Model file for the job. Use its own axes, mm. A direction names the side the tool comes from. Give positions to 0.01 mm unless a question says otherwise; leave off trailing zeros. Order: outer loops, then holes, each group sorted by start corner. A loop starts at its lowest first (then second) coordinate and runs counter-clockwise, first axis right, second up. Notation, with made-up numbers: (81, 0.5) -> (102, 0.5) arc R5 cw to (102, 9.5) -> close; hole circle Ø5 at (41.5, -37). An arc over 180 degrees is marked (long way). Answer in a Markdown table with one row per item. Add a question column.
Autodesk Inventor part; units mm, degrees
ref_plane "Work Plane1" through (0, 0, 18.4) normal (0, 0, -1) x (-1, 0, 0)
ref_plane "YZ Plane" through (0, 0, 0) normal (1, 0, 0) x (0, 1, 0)
ref_plane "XZ Plane" through (0, 0, 0) normal (0, 1, 0) x (-1, 0, 0)
sketch "Sketch1" plane through (0, 0, 0) normal (0, 0, 1) x (1, 0, 0)
  line L0 (-11.5182, 8.1773) -> (10.9818, 8.1773)
  line L1 (10.9818, 8.1773) -> (10.9818, -3.6227)
  line L2 (10.9818, -3.6227) -> (-11.5182, -3.6227)
  line L3 (-11.5182, -3.6227) -> (-11.5182, 8.1773)
  point P0 (0, 0)
  dimension "d0" = 22.5
  dimension "d1" = 11.8
extrude "Extrusion1" add sketch "Sketch1" along normal blind 22.7
sketch "Sketch2" plane through (0, 0, 22.7) normal (0, 0, 1) x (1, 0, 0)
  arc A0 (-0.2741, 4.7773) -> (-0.2741, -0.2227) centre (-5.6182, 2.2773) ccw
  line L0 (-11.5182, 8.1773) -> (-11.5182, -3.6227)
  line L1 (-11.5182, -3.6227) -> (10.9818, -3.6227)
  line L2 (-0.2741, 4.7773) -> (0.6818, 4.7773)
  line L3 (0.6818, -0.2227) -> (-0.2741, -0.2227)
  arc A1 (0.6818, -0.2227) -> (0.6818, 4.7773) centre (0.6818, 2.2773) ccw
  line L4 (3.1818, 2.2773) -> (3.1818, 4.4746) construction
  point P0 (0, 0)
  dimension "d4" = 11.8
  dimension "d5" = 5.9
  dimension "d6" = 5
  dimension "d7" = 8.8
  dimension "d8" = 2.5
extrude "Extrusion2" add sketch "Sketch2" along normal blind 4 contours L2 A1 L3 A0
sketch "Sketch3" plane through (0, 0, 26.7) normal (0, 0, 1) x (1, 0, 0)
  line L0 (0.6818, 4.7773) -> (-0.2741, 4.7773)
  arc A0 (-0.2741, 4.7773) -> (-0.2741, -0.2227) centre (-5.6182, 2.2773) ccw
  line L1 (-0.2741, -0.2227) -> (0.6818, -0.2227)
  arc A1 (0.6818, -0.2227) -> (0.6818, 4.7773) centre (0.6818, 2.2773) ccw
  circle A2 centre (-5.6182, 2.2773) radius 2.3
  point P0 (0, 0)
  dimension "d11" = 4.6
extrude "Extrusion3" add sketch "Sketch3" along normal blind 3.2 contours A2
ref_plane "Work Plane1" through (0, 0, 18.4) normal (0, 0, -1) x (-1, 0, 0)
sketch "Sketch4" plane through (0, 0, 18.4) normal (0, 0, -1) x (-1, 0, 0)
  line L0 (11.5182, 8.1773) -> (-10.9818, 8.1773)
  line L1 (-10.9818, 8.1773) -> (-10.9818, -3.6227)
  line L2 (-10.9818, -3.6227) -> (11.5182, -3.6227)
  line L3 (11.5182, -3.6227) -> (11.5182, 8.1773)
  line L4 (11.5182, 8.1773) -> (16.2182, 8.1773)
  line L5 (16.2182, 8.1773) -> (16.2182, -3.6227)
  line L6 (16.2182, -3.6227) -> (11.5182, -3.6227)
  line L7 (11.5182, -3.6227) -> (11.5182, 8.1773)
  line L8 (-10.9818, 8.1773) -> (-15.6818, 8.1773)
  line L9 (-15.6818, 8.1773) -> (-15.6818, -3.6227)
  line L10 (-15.6818, -3.6227) -> (-10.9818, -3.6227)
  line L11 (-10.9818, -3.6227) -> (-10.9818, 8.1773)
  arc A0 (14.6782, 2.9273) -> (14.6782, 1.6273) centre (13.9182, 2.2773) ccw
  arc A1 (-14.1417, 1.6273) -> (-14.1417, 2.9273) centre (-13.3818, 2.2773) ccw
  line L12 (-14.1417, 2.9273) -> (-15.6818, 2.9273)
  line L13 (-14.1417, 1.6273) -> (-15.6818, 1.6273)
  line L14 (16.2182, 2.9273) -> (14.6782, 2.9273)
  line L15 (16.2182, 1.6273) -> (14.6782, 1.6273)
  point P0 (0, 0)
  dimension "d15" = 4.7
  dimension "d16" = 4.7
  dimension "d17" = 5.9
  dimension "d18" = 5.9
  dimension "d19" = 2
  dimension "d20" = 2
  dimension "d23" = 2.3
  dimension "d24" = 2.3
  dimension "d25" = 1.3
  dimension "d26" = 1.3
  dimension "d27" = 0.65
  dimension "d28" = 0.65
extrude "Extrusion4" add sketch "Sketch4" along normal blind 2.5 contours L4 L5 L14 A0 L15 L6 L3 | L1 L10 L9 L13 A1 L12 L8
sketch "Sketch5" plane through (-11.5182, -3.6227, 0) normal (-1, 0, 0) x (0, 0, 1)
  line L0 (5.7, 7.7) -> (4.5, 7.7)
  line L1 (4.5, 7.7) -> (4.5, 4.1)
  line L2 (4.5, 4.1) -> (5.7, 4.1)
  line L3 (5.7, 4.1) -> (5.7, 7.7)
  line L4 (0, 0) -> (0, 11.8)
  line L5 (0, 5.9) -> (2.0483, 5.9) construction
  point P0 (0, 3.6227)
  dimension "d31" = 1.2
  dimension "d32" = 3.6
  dimension "d33" = 4.5
fillet "Fillet1" radius 0.25 4 edges at (-11.5182, 2.2773, 26.7) (0.2038, 4.7773, 26.7) (0.2038, -0.2227, 26.7) (3.1818, 2.2773, 26.7)
sketch "Sketch6" plane through (-11.5182, -3.6227, 0) normal (-1, 0, 0) x (0, 0, 1)
  arc A0 (5.2906, 6.4417) -> (4.8906, 6.4417) centre (5.0906, 6.9) ccw
  line L0 (4.8816, 4.4457) -> (5.2851, 7.2539) construction
  line L1 (5.2906, 6.4417) -> (5.2906, 6.3583)
  line L2 (5.2906, 5.4417) -> (5.2906, 5.3583)
  arc A1 (4.8906, 5.3583) -> (5.2906, 5.3583) centre (5.0906, 4.9) ccw
  arc A2 (5.2906, 5.4417) -> (5.2906, 6.3583) centre (5.0906, 5.9) ccw
  arc A3 (4.8906, 6.3583) -> (4.8906, 5.4417) centre (5.0906, 5.9) ccw
  line L3 (5.2906, 3.9094) -> (5.0683, 6.1222) construction
  line L4 (4.8787, 7.3529) -> (4.8906, 7.2532) construction
  line L5 (4.8906, 5.3583) -> (4.8906, 5.4417)
  line L6 (4.8906, 6.3583) -> (4.8906, 6.4417)
  line L7 (0, 0) -> (0, 11.8)
  point P0 (0, 3.6227)
  point P1 (0, 5.9)
  dimension "d39" = 1
  dimension "d40" = 2
  dimension "d42" = 0.4
  dimension "d43" = 0.4
  dimension "d44" = 5.0906
  dimension "d45" = 0.5
  dimension "d46" = 0.5
  dimension "d47" = 0.5
  dimension "d48" = 1
  dimension "d49" = 1
  dimension "d50" = 0.2
  dimension "d51" = 0.2
  dimension "d52" = 0.2
  dimension "d53" = 0.5
  dimension "d54" = 0.2
sketch "Sketch7" plane through (-5.6182, 2.2773, 29.9) normal (0, 0, 1) x (1, 0, 0)
  circle A0 centre (0, 0) radius 0.5
  point P0 (5.6182, -2.2773)
  dimension "d55" = 1
extrude "Extrusion6" cut sketch "Sketch7" against normal blind 3
fillet "Fillet2" radius 0.5 4 edges at (10.9818, 8.1773, 7.95) (-11.5182, 8.1773, 7.95) (-11.5182, -3.6227, 7.95) (10.9818, -3.6227, 7.95)
properties part number "servo motor"
Item 1: Wall check: line 1 (X direction, y = 3.25, z = 9); line 2 (Z direction, x = 14.5, y = 6.75); line 3 (Z direction, x = -7, y = -1.5). Give the ranges that are in metal, low to high.
Item 2: Saw through at A-A on z = 2.25. List the corners of the cut face in (x, y), plus the area to 3 significant figures.
Item 3: Saw through at D-D on z = 21.75. List the corners of the cut face in (x, y).
Item 4: Saw through at B-B on x = 4. List the corners of the cut face in (y, z).
Item 5: Saw through at C-C on z = 28.25. List the corners of the cut face in (x, y), plus the area to 3 significant figures.
Item 6: Which spindle directions (+Z, -Z, +X, -X, +Y, -Y) get a long thin tool onto all of the face, cutting with end or side? Do faces 4 (the flat face through (0, 4.777, 25)), 5 (the flat face through (10.982, 2, 21)), 6 (the flat face through (-11.518, 2, 8)), 7 (the cylindrical face through (-6.12, 4.52, 28.28)), 8 (the flat face through (-10, -2, 22.7)). Say none if no direction does.
Item 7: Two-plate mould, pull along Y, no slides. Class faces 1 (the cylindrical face through (3.18, 2.33, 24.55)), 2 (the flat face through (-3, 2, 26.7)), 3 (the flat face through (15, 2.927, 17)): pulls with the +Y half, pulls with the -Y half, needs draft (parallel to the pull), parting line crosses it, or undercut.
Item 8: Pin check, flat tips, straight feed: pin 1 Ø1.6 at (x, y) = (-14.5, 4.5) entering from -Z; pin 2 Ø1.5 at (y, z) = (-2, 24) entering from +X; pin 3 Ø5.5 at (y, z) = (1.5, 11) entering from -X. Stop position of each tip, or through.
Evaluation:
| question | item | result |
|---|---|---|
| 1 | line 1 | x = -11.52 to 10.98 |
| 1 | line 2 | z = 15.9 to 18.4 |
| 1 | line 3 | z = 0 to 26.7 |
| 2 | outline | (-11.52, -3.12) arc R0.5 ccw to (-11.02, -3.62) -> (10.48, -3.62) arc R0.5 ccw to (10.98, -3.12) -> (10.98, 7.68) arc R0.5 ccw to (10.48, 8.18) -> (-11.02, 8.18) arc R0.5 ccw to (-11.52, 7.68) -> close |
| 2 | area | 265 mm2 |
| 3 | outline | (-11.52, -3.62) -> (10.98, -3.62) -> (10.98, 8.18) -> (-11.52, 8.18) -> close |
| 4 | outline | (-3.62, 0) -> (8.18, 0) -> (8.18, 22.7) -> (-3.62, 22.7) -> close |
| 5 | outline | circle Ø4.6 at (-5.62, 2.28); hole circle Ø1 at (-5.62, 2.28) |
| 5 | area | 15.8 mm2 |
| 6 | face 4 | +Z, +X, +Y |
| 6 | face 5 | +Z, +X, +Y, -Y |
| 6 | face 6 | -Z, -X, +Y, -Y |
| 6 | face 7 | +Z |
| 6 | face 8 | +Z, -X, -Y |
| 7 | face 1 | parting line crosses it |
| 7 | face 2 | needs draft |
| 7 | face 3 | undercut |
| 8 | pin 1 | stops at z = 15.9 |
| 8 | pin 2 | stops at x = -0.89 |
| 8 | pin 3 | stops at x = -11.52 |
